Read the model definition and answer for the solid it produces. Units are mm, in the model's axes. A direction names the side the tool comes from. Coordinates: 2 decimals unless noted, no trailing zeros. Loops run counter-clockwise (first coordinate to the right, second up) from the corner with the lowest first, then second, coordinate; pieces in that order, holes last. Notation, with made-up numbers: (27, 74) - (75, 74) arc R10 cw to (75, 79) - close; hole circle Ø7 at (30, 24.5). An arc over 180 degrees is marked (long way). Use one line per item in the form item = value.
from build123d import *

# Parameters (mm, degrees)
F1_DEPTH = 50
F2_SIZE2 = 1
F2_SIZE  = 5
F3_SIZE2 = 5
F3_SIZE  = 1
F5_DEPTH = 25


with BuildPart() as f1:
    # F0 (on Front) → F1 (new body)
    with BuildSketch(Plane.XZ):
        Polygon((40.5, 0), (0, 0), (0, 2), (-3, 2), (-3, -6), (0, -6), (40.5, -6), (43.5, -6), (43.5, 2), (40.5, 2), align=None)
    extrude(amount=F1_DEPTH)

    # F2
    f2_edges = [f1.edges().sort_by_distance(p)[0] for p in [
        (-3, -25, 2),
    ]]
    f2_side = f1.faces().sort_by_distance((-3, -25, -2))[0]
    chamfer(f2_edges, length=F2_SIZE, length2=F2_SIZE2, reference=f2_side)

    # F3
    f3_edges = [f1.edges().sort_by_distance(p)[0] for p in [
        (43.5, -25, 2),
    ]]
    f3_side = f1.faces().sort_by_distance((42, -25, 2))[0]
    chamfer(f3_edges, length=F3_SIZE, length2=F3_SIZE2, reference=f3_side)

    # F4 (on face) → F5 (cut)
    with BuildSketch(Plane.XY):
        with BuildLine():
            ThreePointArc((30.5, -35), (32.267766953, -34.267766953), (33, -32.5))
            Line((33, -32.5), (33, -17.5))
            ThreePointArc((33, -17.5), (32.267766953, -15.732233047), (30.5, -15))
            ThreePointArc((30.5, -15), (28.732233047, -15.732233047), (28, -17.5))
            Line((28, -17.5), (28, -32.5))
            ThreePointArc((28, -32.5), (28.732233047, -34.267766953), (30.5, -35))
        make_face()
    extrude(amount=-F5_DEPTH, mode=Mode.SUBTRACT)


solid = f1.part
Item 1: Find the intervals of material crossed by L1, parallel to X at y = -21.5, z = -3.5; L2, parallel to Z at x = 28, y = -17; L3, parallel to X at y = -34.5, z = -2, in increasing order.
Results below:
L1 = -3 to 28, 33 to 43.5
L2 = -6 to 0
L3 = -2.8 to 29, 32 to 43.3
Item 2: The part is cut by section B-B on z = -2.25. Give the vertices of the cut face in (x, y).
Results below:
outline = (-2.85, -50) - (43.35, -50) - (43.35, 0) - (-2.85, 0) - close; hole (28, -32.5) arc R2.5 ccw to (33, -32.5) - (33, -17.5) arc R2.5 ccw to (28, -17.5) - close
Item 3: The part is cut by section D-D on y = -11. Give the vertices of the cut face in (x, z), plus the area to 3 significant figures.
Results below:
outline = (-3, -6) - (43.5, -6) - (43.5, -3) - (42.5, 2) - (40.5, 2) - (40.5, 0) - (0, 0) - (0, 2) - (-2, 2) - (-3, -3) - close
area = 286 mm²
Item 4: Which of the six approach directions +Z, -Z, +X, -X, +Y, -Y give full straight-line access (tool end or side, diameter ignored) to faces 4 (the flat face through (40.5, -25, 1)), 5 (the flat face through (33, -25, -3)), 6 (the flat face through (-2.5, -24.7, -0.5))?
Results below:
face_4 = +Z, +Y, -Y
face_5 = +Z, -Z
face_6 = +Z, -X, +Y, -Y
Item 5: The part is cut by section A-A on y = -25. Give the vertices of the cut face in (x, z), plus the area to 3 significant figures.
Results below:
outline = (-3, -6) - (28, -6) - (28, 0) - (0, 0) - (0, 2) - (-2, 2) - (-3, -3) - close; (33, -6) - (43.5, -6) - (43.5, -3) - (42.5, 2) - (40.5, 2) - (40.5, 0) - (33, 0) - close
area = 256 mm²
Item 6: For a pull along Y with two mould halves and no side action, classify faces 1 (the flat face through (20, 0, -3)), 2 (the flat face through (21, -25, 0)), 3 (the flat face through (28, -25, -3)) as +Y half, -Y half, draft (parallel to the pull), parting line (faces both ways), or undercut.
Results below:
face_1 = +Y half
face_2 = draft
face_3 = undercut
Item 7: The part is cut by section C-C on z = 1. Give the vertices of the cut face in (x, y), plus the area to 3 significant figures.
Results below:
outline = (-2.2, -50) - (0, -50) - (0, 0) - (-2.2, 0) - close; (40.5, -50) - (42.7, -50) - (42.7, 0) - (40.5, 0) - close
area = 220 mm²
Item 8: Each of these flat-tipped pins is pushed along its axis until it touches: P1, Ø0.6, axis at y = -35.5, z = 1.5, coming from the +X side; P2, Ø2, axis at y = -9.5, z = -1, coming from the +X side; P3, Ø0.6, axis at y = -34.5, z = 1, coming from the -X side. Where does it stop, or does it pass through?
Results below:
P1 = 42.66
P2 = 43.3
P3 = -2.26
